Read the model definition and answer for the solid it produces. Units are mm, in the model's axes. Face numbers are marked on the shaded views. A direction names the side the tool comes from. Coordinates: 2 decimals unless noted, no trailing zeros. Order: outer loops, then holes, each group sorted by start corner. A loop starts at its lowest first (then second) coordinate and runs counter-clockwise, first axis right, second up. Notation, with made-up numbers: (-12.5, 34) -> (-7.5, 34) arc R27 ccw to (-7.5, 66) -> close; hole circle Ø2 at (-32.75, 85.25). An arc over 180 degrees is marked (long way). Answer in a Markdown table with one row per item.
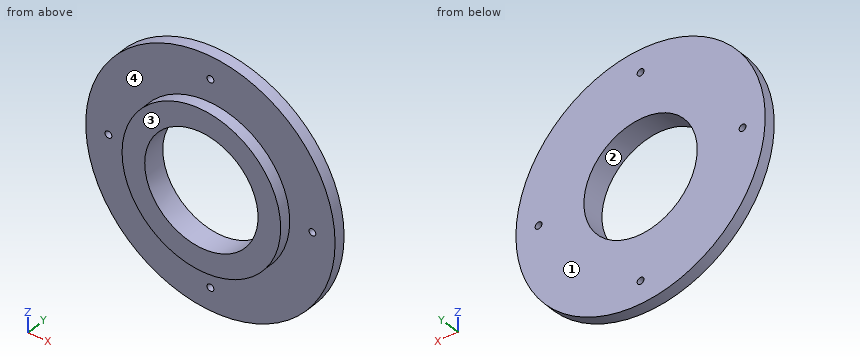
from build123d import *

# Parameters (mm, degrees)
F0_R     = 55
F1_DEPTH = 5
F2_R     = 35
F3_DEPTH = 5
F4_R     = 25
F5_DEPTH = 25
F6_R     = 1.5
F7_DEPTH = 12


with BuildPart() as f1:
    # F0 (on Front) → F1 (new body)
    with BuildSketch(Plane.XZ):
        Circle(F0_R)
    extrude(amount=F1_DEPTH)

    # F2 (on face) → F3 (join)
    with BuildSketch(Plane.XZ.offset(5)):
        Circle(F2_R)
    extrude(amount=F3_DEPTH)

    # F4 (on face) → F5 (cut)
    with BuildSketch(Plane(origin=(0, 0, 0), x_dir=(-1, 0, 0), z_dir=(0, 1, 0))):
        Circle(F4_R)
    extrude(amount=-F5_DEPTH, mode=Mode.SUBTRACT)

    # F6 (on face) → F7 (cut)
    with BuildSketch(Plane.XZ.offset(10)):
        with Locations((-45, 0)):
            Circle(F6_R)
        with Locations((0, 45)):
            Circle(F6_R)
        with Locations((0, -45)):
            Circle(F6_R)
        with Locations((45, 0)):
            Circle(F6_R)
    extrude(amount=-F7_DEPTH, mode=Mode.SUBTRACT)


solid = f1.part
Q1. Consider line 1 (Z direction, x = 0, y = -3); line 2 (Z direction, x = 45, y = -3.6); line 3 (X direction, y = -5.25, z = 10.5). Determine where each line is inside the solid, lowest interval first.
Outcome:
| item | result |
|---|---|
| line 1 | -55 to -46.5, -43.5 to -25, 25 to 43.5, 46.5 to 55 |
| line 2 | -31.62 to -1.5, 1.5 to 31.62 |
| line 3 | -33.39 to -22.69, 22.69 to 33.39 |
Q2. For the marked faces 3 and 4, determine the directions among +Z, -Z, +X, -X, +Y, -Y from which every point of the face is accessible in a straight line to the end or side of a thin tool.
Outcome:
| item | result |
|---|---|
| face 3 | +Z, -Z, +X, -X, -Y |
| face 4 | -Y |
Q3. The part is cut by section D-D (z = 18). Write down the section's boundary in (x, y), then the cut area to 3 significant figures.
Outcome:
| item | result |
|---|---|
| outline | (-51.97, -5) -> (-30.02, -5) -> (-30.02, -10) -> (-17.35, -10) -> (-17.35, 0) -> (-51.97, 0) -> close; (17.35, -10) -> (30.02, -10) -> (30.02, -5) -> (51.97, -5) -> (51.97, 0) -> (17.35, 0) -> close |
| area | 473 mm² |
Q4. Given pin 1 (5 mm diameter, centred on x = 44, y = -1.5, fed in from -Z); pin 2 (2.5 mm diameter, centred on x = 45, z = 0, fed in from +Y); pin 3 (2 mm diameter, centred on x = -37, z = -16, fed in from +Y); pin 4 (3.5 mm diameter, centred on x = 0, z = -45, fed in from -Y), each flat-ended and moving along its own axis, determine where each tip first touches the part or whether it passes through.
Outcome:
| item | result |
|---|---|
| pin 1 | z = -36.09 |
| pin 2 | through |
| pin 3 | y = 0 |
| pin 4 | y = -5 |
Q5. For a pull along Z with two mould halves and no side action, classify the marked faces 1 and 2 as pulls with the +Z half, pulls with the -Z half, needs draft (parallel to the pull), parting line crosses it, or undercut.
Outcome:
| item | result |
|---|---|
| face 1 | needs draft |
| face 2 | undercut |
Q6. The part is cut by section C-C (x = 17). Write down the section's boundary in (y, z).
Outcome:
| item | result |
|---|---|
| outline | (-10, -30.59) -> (-5, -30.59) -> (-5, -52.31) -> (0, -52.31) -> (0, -18.33) -> (-10, -18.33) -> close; (-10, 18.33) -> (0, 18.33) -> (0, 52.31) -> (-5, 52.31) -> (-5, 30.59) -> (-10, 30.59) -> close |
Q7. The part is cut by section B-B (y = -3.75). Write down the section's boundary in (x, z).
Outcome:
| item | result |
|---|---|
| outline | circle Ø110 at (0, 0); hole circle Ø3 at (-45, 0); hole circle Ø50 at (0, 0); hole circle Ø3 at (0, -45); hole circle Ø3 at (0, 45); hole circle Ø3 at (45, 0) |
Q8. The part is cut by section A-A (x = 0). Write down the section's boundary in (y, z), then the cut area to 3 significant figures.
Outcome:
| item | result |
|---|---|
| outline | (-10, -35) -> (-5, -35) -> (-5, -43.5) -> (0, -43.5) -> (0, -25) -> (-10, -25) -> close; (-10, 25) -> (0, 25) -> (0, 43.5) -> (-5, 43.5) -> (-5, 35) -> (-10, 35) -> close; (-5, -55) -> (0, -55) -> (0, -46.5) -> (-5, -46.5) -> close; (-5, 46.5) -> (0, 46.5) -> (0, 55) -> (-5, 55) -> close |
| area | 370 mm² |
